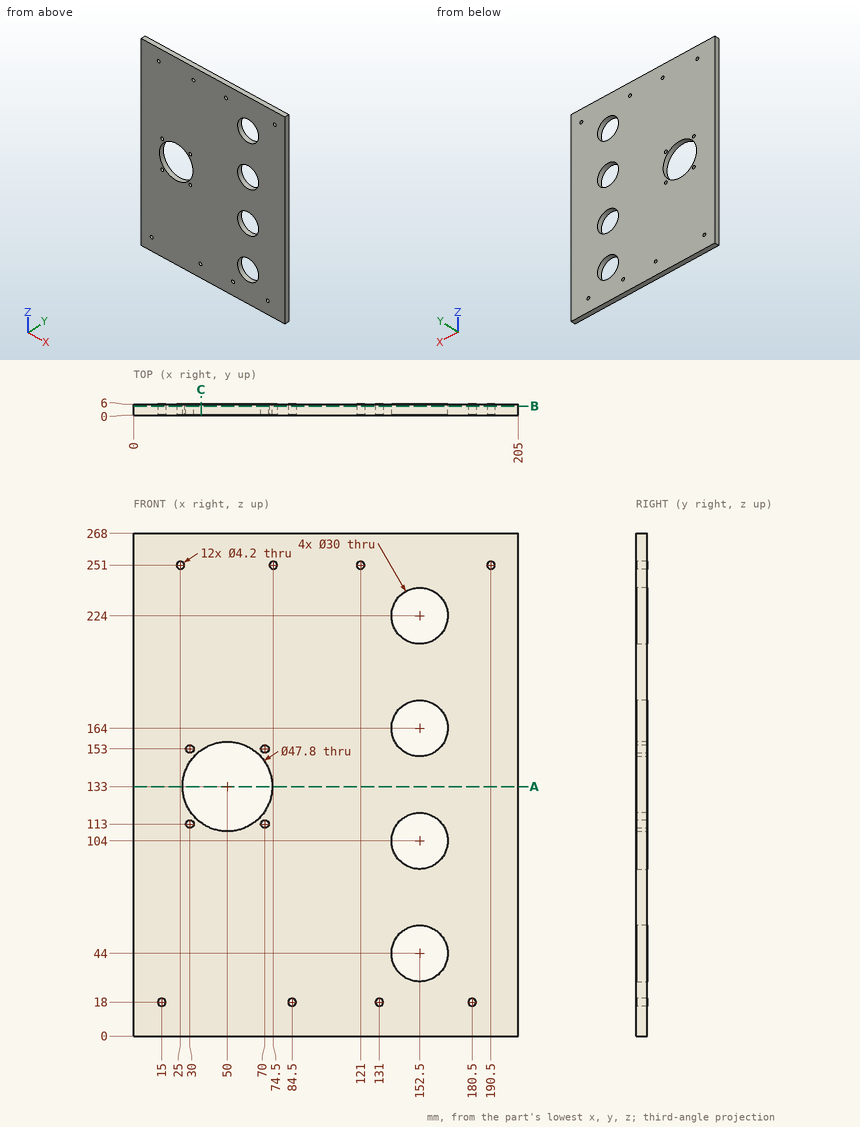
Answer from the drawing. Dimensions are ordinates in mm from the lowest x, y and z of the part. Coordinates: 2 decimals unless noted, no trailing zeros. Loops run counter-clockwise (first coordinate to the right, second up) from the corner with the lowest first, then second, coordinate; pieces in that order, holes last. Notation, with made-up numbers: (-5, 30.5) - (7, 30.5) arc R17 ccw to (7, 55.5) - close; hole circle Ø10 at (78, 66). An arc over 180 degrees is marked (long way). Answer in a Markdown table with one row per item.
1. Given pin 1 (8 mm diameter, centred on x = 46.5, z = 110.5, fed in from +Y), flat-ended and moving along its own axis, determine where the tip first touches the part or whether it passes through.
Conclusion:
| item | result |
|---|---|
| pin 1 | stops at y = 6 |
2. Find section B-B, the plane y = 4.8. Count the separate pieces of the cut face and the enclosed holes in it, then the cut area to 3 significant figures.
Conclusion:
| item | result |
|---|---|
| separate pieces | 1 |
| enclosed holes | 17 |
| area | 50,200 mm² |
3. Find section A-A, the plane z = 133. Write down the section's boundary in (x, y).
Conclusion:
| item | result |
|---|---|
| outline | (0, 0) - (26.1, 0) - (26.1, 6) - (0, 6) - close; (73.9, 0) - (205, 0) - (205, 6) - (73.9, 6) - close |
4. Straight lines are drawn through the part: line 1 (X direction, y = 3.9, z = 18); line 2 (Z direction, x = 84.5, y = 3.75); line 3 (X direction, y = 4.3, z = 113). For each, find the intervals that lie inside material, in ascending order.
Conclusion:
| item | result |
|---|---|
| line 1 | x = 0 to 12.9, 17.1 to 82.4, 86.6 to 128.9, 133.1 to 178.4, 182.6 to 205 |
| line 2 | z = 0 to 15.9, 20.1 to 268 |
| line 3 | x = 0 to 27.9, 32.1 to 36.92, 63.08 to 67.9, 72.1 to 140.5, 164.5 to 205 |
5. Find section C-C, the plane x = 36. Write down the section's boundary in (y, z).
Conclusion:
| item | result |
|---|---|
| outline | (0, 0) - (6, 0) - (6, 113.63) - (0, 113.63) - close; (0, 152.37) - (6, 152.37) - (6, 268) - (0, 268) - close |
